Read the model definition and answer for the solid it produces. Units are mm, in the model's axes. Face numbers are marked on the shaded views. A direction names the side the tool comes from. Coordinates: 2 decimals unless noted, no trailing zeros. Write each loop counter-clockwise with the first axis right and the second up, starting at its lowest first coordinate (ties: lowest second). Pieces come first, ordered by that corner, then holes. Notation, with made-up numbers: (27.5, 73) -> (45.5, 73) arc R15 cw to (45.5, 80) -> close; hole circle Ø1 at (17, 10). An arc over 180 degrees is marked (long way). Return JSON: item names as keys, results as strings.
from build123d import *

# Parameters (mm, degrees)
SKETCH_1_W               = 100
SKETCH_1_H               = 100
EXTRUDE_1_DEPTH          = 100
EXTRUDE_2_DEPTH          = 5
SKETCH_4_W               = 100
SKETCH_4_H               = 100
EXTRUDE_3_DEPTH          = 3
PATTERN_CIRCULAR_1_COUNT = 4
SKETCH_7_R               = 15
SKETCH_7_R_2             = 13
EXTRUDE_5_DEPTH          = 20
SKETCH_8_R               = 7.5
SKETCH_8_R_2             = 6
EXTRUDE_6_DEPTH          = 15
SKETCH_11_R              = 7.210019968
CUT_EXTRUDE_2_DEPTH      = 5


with BuildPart() as part:
    # Эскиз1 → Бобышка-Вытянуть1 (new body)
    with BuildSketch(Plane(origin=(0, 0, 0), x_dir=(1, 0, 0), z_dir=(0, 1, 0))):
        Rectangle(SKETCH_1_W, SKETCH_1_H)
    extrude(amount=EXTRUDE_1_DEPTH)

    # Эскиз3 → Бобышка-Вытянуть2 (add, symmetric)
    with BuildSketch(Plane.XY):
        Polygon((60, -10), (60, -15), (45, -15), (45, 0), (50, 0), (50, -10), align=None)
    extrude_2 = extrude(amount=EXTRUDE_2_DEPTH, both=True)

    # Эскиз4 → Бобышка-Вытянуть3 (add)
    with BuildSketch(Plane.XZ.offset(15)):
        with Locations((110, 0)):
            Rectangle(SKETCH_4_W, SKETCH_4_H)
    extrude_3 = extrude(amount=-EXTRUDE_3_DEPTH)

    # Круговой массив1: Бобышка-Вытянуть2, Бобышка-Вытянуть3 ×4 about axis
    pattern_circular_1_axis = Axis((0, 0, 0), (0, 1, 0))
    for i in range(1, PATTERN_CIRCULAR_1_COUNT):
        add(extrude_2.rotate(pattern_circular_1_axis, i * 360 / PATTERN_CIRCULAR_1_COUNT))
        add(extrude_3.rotate(pattern_circular_1_axis, i * 360 / PATTERN_CIRCULAR_1_COUNT))

    # Эскиз7 → Бобышка-Вытянуть5 (add)
    with BuildSketch(Plane(origin=(0, 100, 0), x_dir=(1, 0, 0), z_dir=(0, 1, 0))):
        with Locations((-30, -30)):
            Circle(SKETCH_7_R)
        with Locations((-30, -30)):
            Circle(SKETCH_7_R_2, mode=Mode.SUBTRACT)
    extrude(amount=EXTRUDE_5_DEPTH)

    # Эскиз8 → Бобышка-Вытянуть6 (add)
    with BuildSketch(Plane(origin=(0, 100, 0), x_dir=(1, 0, 0), z_dir=(0, 1, 0))):
        with Locations((40, 40)):
            Circle(SKETCH_8_R)
        with Locations((40, 40)):
            Circle(SKETCH_8_R_2, mode=Mode.SUBTRACT)
    extrude(amount=EXTRUDE_6_DEPTH)

    # Эскиз10 → Повернуть1 (revolve)
    with BuildSketch(Plane.XY):
        with BuildLine():
            Line((8.680645457, 130.445795914), (7.680645457, 130.445795914))
            add(Edge.make_bspline(
                [(7.680645457, 130.445795914), (7.680645457, 127.036197798), (1.669418546, 117.303060729), (8.436480148, 106.717484225), (8.436480148, 100)],
                knots=[0, 0, 0, 0, 0.331036339, 1, 1, 1, 1], degree=3))
            Line((8.436480148, 100), (9.436480148, 100))
            add(Edge.make_bspline(
                [(8.680645457, 130.445795914), (8.680645457, 129.743031745), (8.522630114, 128.322957752), (7.990188694, 126.341389545), (7.322411145, 124.435424215), (6.663640941, 122.600134826), (6.143869676, 120.828668813), (5.810471482, 118.538078927), (6.008246237, 115.536453962), (6.892964845, 111.786431822), (8.442762115, 106.643818661), (9.436480148, 102.680139866), (9.436480148, 100)],
                knots=[0, 0, 0, 0, 0.0625, 0.125, 0.1875, 0.25, 0.3125, 0.375, 0.5, 0.625, 0.75, 1, 1, 1, 1], degree=3))
        make_face()
    revolve(axis=Axis((0, 100, 0), (0, 1, 0)))

    # Эскиз11 → Вырез-Вытянуть2 (cut)
    with BuildSketch(Plane.XZ):
        with Locations((-26.927393067, 25.615882257)):
            Circle(SKETCH_11_R)
    extrude(amount=-CUT_EXTRUDE_2_DEPTH, mode=Mode.SUBTRACT)


solid = part.part
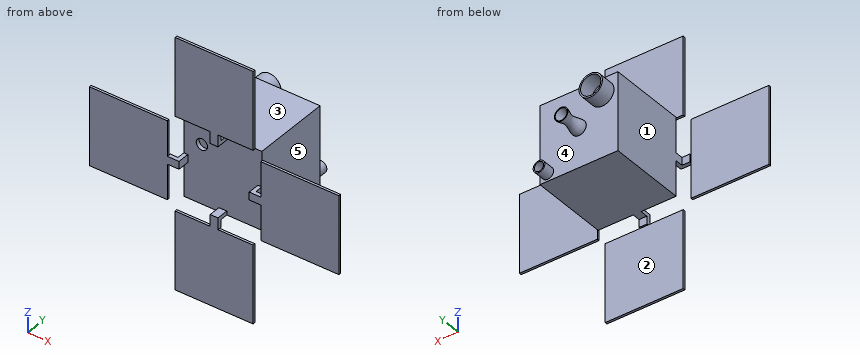
1. The part is cut by section D-D (y = 70). Determine the outline of the cut face in (x, z).
Taken from the geometry:
{"outline": "(-50, -50) -> (50, -50) -> (50, 50) -> (-50, 50) -> close"}
2. The part is cut by section A-A (z = -40). Determine the outline of the cut face in (x, y), then the cut area to 3 significant figures.
Taken from the geometry:
{"outline": "(-160, -15) -> (-60, -15) -> (-60, -12) -> (-160, -12) -> close; (-50, 0) -> (50, 0) -> (50, 100) -> (47.5, 100) -> (47.5, 115) -> (46, 115) -> (46, 100) -> (34, 100) -> (34, 115) -> (32.5, 115) -> (32.5, 100) -> (-50, 100) -> close; (60, -15) -> (160, -15) -> (160, -12) -> (60, -12) -> close", "area": "10,600 mm2"}
3. A tool of negligible diameter and unlimited length cuts with its end or side. For the marked faces 1, 2, 3, 4 and 5, from which of +Z, -Z, +X, -X, +Y, -Y can it reach the whole face along a straight path? Write none if from no direction.
Taken from the geometry:
{"face 1": "+Z, -Z, -X, +Y", "face 2": "-Z, +X, -X, +Y", "face 3": "+Z, +X, -X, +Y", "face 4": "+Y", "face 5": "+Z, -Z, +X, +Y"}
4. Flat-ended cylindrical pins translate along their axes: pin 1 Ø0.9 at (y, z) = (-13, -115.5) entering from -X; pin 2 Ø3 at (x, y) = (-1, -5) entering from -Z; pin 3 Ø8 at (y, z) = (57, -19.5) entering from +X. Find the tip coordinate at first contact, or state that the pin passes through.
Taken from the geometry:
{"pin 1": "stops at x = -50", "pin 2": "stops at z = -50", "pin 3": "stops at x = 50"}
5. The part is cut by section B-B (x = -30). Determine the outline of the cut face in (y, z), then the cut area to 3 significant figures.
Taken from the geometry:
{"outline": "(-15, -160) -> (-12, -160) -> (-12, -60) -> (-15, -60) -> close; (-15, 60) -> (-12, 60) -> (-12, 160) -> (-15, 160) -> close; (0, -50) -> (100, -50) -> (100, 15) -> (120, 15) -> (120, 17) -> (100, 17) -> (100, 43) -> (120, 43) -> (120, 45) -> (100, 45) -> (100, 50) -> (0, 50) -> (0, 32.14) -> (5, 32.14) -> (5, 19.09) -> (0, 19.09) -> close", "area": "10,600 mm2"}
6. Consider L1, parallel to X at y = 113, z = 30; L2, parallel to Z at x = -30, y = 112; L3, parallel to Y at x = -17.5, z = 68.5. Determine where each line is inside the solid, lowest interval first.
Taken from the geometry:
{"L1": "x = -45 to -43, -17 to -15", "L2": "z = 15 to 17, 43 to 45", "L3": "y = -15 to -12"}
7. The part is cut by section C-C (z = -133). Determine the outline of the cut face in (x, y).
Taken from the geometry:
{"outline": "(-50, -15) -> (50, -15) -> (50, -12) -> (-50, -12) -> close"}
